Can you work these out from the model? Positions are in its coordinate system, mm. A direction names the side the tool comes from. Give positions to 0.01 mm unless a question says otherwise; leave off trailing zeros. Order: outer loops, then holes, each group sorted by start corner. A loop starts at its lowest first (then second) coordinate and runs counter-clockwise, first axis right, second up. Notation, with made-up numbers: (-10, -3) - (10, -3) arc R35 cw to (10, 32) - close; hole circle Ø8 at (-10.5, 82.5). An arc over 180 degrees is marked (long way). Answer as a JSON object with one key per item and string values.
```python
from build123d import *

# Parameters (mm, degrees)
F0_W      = 155
F0_H      = 80.5
F1_DEPTH  = 8.6
F2_T      = -1.5
F3_W      = 155
F3_H      = 80.5
F3_W_2    = 152
F3_H_2    = 77.5
F3_W_3    = 149
F3_H_3    = 74.5
F4_DEPTH  = 1.5
F5_W      = 28
F5_H      = 7.1
F6_DEPTH  = 1.5
F7_W      = 20
F7_H      = 7.1
F8_DEPTH  = 1.5
F9_R      = 3
F10_DEPTH = 1.5
F11_W     = 38
F11_H     = 6.2492947091
F12_DEPTH = 1.5
F13_W     = 8.8
F13_H     = 4.4
F13_W_2   = 15.4
F13_H_2   = 7.7
F14_DEPTH = 1.5
F15_R     = 1.5
F16_R     = 2
F17_R     = 5
F18_R     = 3
F20_DEPTH = 2
F21_R     = 1.99999
F23_DEPTH = 2
F24_R     = 1.5
F25_DEPTH = 2
F26_R     = 1.5


# Not quite as in the source:
# - a fillet or chamfer is up to 0.001 mm smaller than in the source, because OpenCascade refuses the exact size


with BuildPart() as f1:
    # F0 (on Top) → F1 (new body)
    with BuildSketch(Plane.XY):
        with Locations((77.5, 40.25)):
            Rectangle(F0_W, F0_H)
    extrude(amount=F1_DEPTH)

    # F2
    f2_openings = [f1.faces().sort_by_distance(p)[0] for p in [
        (77.5, 40.25, 8.6),
    ]]
    offset(amount=F2_T, openings=f2_openings)

    # F3 (on face) → F4 (join)
    with BuildSketch(Plane.XY.offset(8.6)):
        with Locations((77.5, 40.25)):
            Rectangle(F3_W, F3_H)
        with Locations((77.5, 40.25)):
            Rectangle(F3_W_2, F3_H_2, mode=Mode.SUBTRACT)
        with Locations((77.5, 40.25)):
            Rectangle(F3_W_2, F3_H_2)
        with Locations((77.5, 40.25)):
            Rectangle(F3_W_3, F3_H_3, mode=Mode.SUBTRACT)
    extrude(amount=F4_DEPTH)

    # F5 (on face) → F6 (cut, through all)
    with BuildSketch(Plane.XZ):
        with Locations((37.5, 5.05)):
            Rectangle(F5_W, F5_H)
    extrude(amount=-F6_DEPTH, mode=Mode.SUBTRACT)

    # F7 (on face) → F8 (cut, through all)
    with BuildSketch(Plane(origin=(0, 80.5, 0), x_dir=(-1, 0, 0), z_dir=(0, 1, 0))):
        with Locations((-48, 5.05)):
            Rectangle(F7_W, F7_H)
    extrude(amount=-F8_DEPTH, mode=Mode.SUBTRACT)

    # F9 (on face) → F10 (cut, through all)
    with BuildSketch(Plane(origin=(0, 0, 0), x_dir=(0, -1, 0), z_dir=(-1, 0, 0))):
        with Locations((-28, 4.5)):
            Circle(F9_R)
    extrude(amount=-F10_DEPTH, mode=Mode.SUBTRACT)

    # F11 (on face) → F12 (cut, through all)
    with BuildSketch(Plane.YZ.offset(155)):
        with Locations((45.2, 4.6246473546)):
            Rectangle(F11_W, F11_H)
    extrude(amount=-F12_DEPTH, mode=Mode.SUBTRACT)

    # F13 (on face) → F14 (cut, through all)
    with BuildSketch(Plane(origin=(0, 0, 0), x_dir=(1, 0, 0), z_dir=(0, 0, -1))):
        with Locations((26.2872223049, -27.05)):
            Rectangle(F13_W, F13_H)
        with Locations((26.2872223049, -22.65)):
            Rectangle(F13_W, F13_H)
        with Locations((26.2872223049, -35.8)):
            Rectangle(F13_W_2, F13_H_2)
        with Locations((26.2872223049, -43.5)):
            Rectangle(F13_W_2, F13_H_2)
        with Locations((26.2872223049, -52.25)):
            Rectangle(F13_W, F13_H)
        with Locations((26.2872223049, -56.65)):
            Rectangle(F13_W, F13_H)
    extrude(amount=-F14_DEPTH, mode=Mode.SUBTRACT)

    # F15
    f15_edges = [f1.edges().sort_by_distance(p)[0] for p in [
        (23.5, 0.75, 8.6),
        (51.5, 0.75, 8.6),
        (51.5, 0.75, 1.5),
        (23.5, 0.75, 1.5),
        (154.25, 26.2, 7.749295),
        (154.25, 26.2, 1.5),
        (154.25, 64.2, 7.749295),
        (154.25, 64.2, 1.5),
        (58, 79.75, 8.6),
        (58, 79.75, 1.5),
        (38, 79.75, 8.6),
        (38, 79.75, 1.5),
        (21.887222, 50.05, 0.75),
    ]]
    fillet(f15_edges, radius=F15_R)

    # F16
    f16_edges = [f1.edges().sort_by_distance(p)[0] for p in [
        (21.887222, 29.25, 0.75),
        (18.587222, 47.35, 0.75),
        (21.887222, 58.85, 0.75),
        (21.887222, 20.45, 0.75),
        (18.587222, 31.95, 0.75),
        (30.687222, 50.05, 0.75),
        (33.987222, 31.95, 0.75),
        (30.687222, 20.45, 0.75),
        (30.687222, 29.25, 0.75),
        (33.987222, 47.35, 0.75),
        (30.687222, 58.85, 0.75),
    ]]
    fillet(f16_edges, radius=F16_R)

    # F17
    f17_edges = [f1.edges().sort_by_distance(p)[0] for p in [
        (0, 0, 5.05),
        (0, 80.5, 5.05),
        (155, 0, 5.05),
        (155, 80.5, 5.05),
    ]]
    fillet(f17_edges, radius=F17_R)

    # F18
    f18_edges = [f1.edges().sort_by_distance(p)[0] for p in [
        (1.5, 79, 5.05),
        (1.5, 1.5, 5.05),
        (153.5, 79, 5.05),
        (153.5, 1.5, 5.05),
    ]]
    fillet(f18_edges, radius=F18_R)

    # F19 (on face) → F20 (join)
    with BuildSketch(Plane(origin=(0, 0, 0), x_dir=(1, 0, 0), z_dir=(0, 0, -1))):
        with BuildLine():
            Line((26.2872223049, -17.0733576864), (12.2872223049, -17.0733576864))
            Line((12.2872223049, -17.0733576864), (12.2872223049, -65.0733576864))
            Line((12.2872223049, -65.0733576864), (26.2872223049, -65.0733576864))
            Line((26.2872223049, -65.0733576864), (26.2872223049, -58.85))
            Line((26.2872223049, -58.85), (23.8872223049, -58.85))
            ThreePointArc((23.8872223049, -58.85), (22.4730087426, -58.2642135624), (21.8872223049, -56.85))
            Line((21.8872223049, -56.85), (21.8872223049, -51.55))
            ThreePointArc((21.8872223049, -51.55), (22.3265621332, -50.4893398282), (23.3872223049, -50.05))
            Line((23.3872223049, -50.05), (26.2872223049, -50.05))
            Line((26.2872223049, -50.05), (26.2872223049, -47.35))
            Line((26.2872223049, -47.35), (20.5872223049, -47.35))
            ThreePointArc((20.5872223049, -47.35), (19.1730087426, -46.7642135624), (18.5872223049, -45.35))
            Line((18.5872223049, -45.35), (18.5872223049, -33.95))
            ThreePointArc((18.5872223049, -33.95), (19.1730087426, -32.5357864376), (20.5872223049, -31.95))
            Line((20.5872223049, -31.95), (26.2872223049, -31.95))
            Line((26.2872223049, -31.95), (26.2872223049, -29.25))
            Line((26.2872223049, -29.25), (23.8872223049, -29.25))
            ThreePointArc((23.8872223049, -29.25), (22.4730087426, -28.6642135624), (21.8872223049, -27.25))
            Line((21.8872223049, -27.25), (21.8872223049, -22.45))
            ThreePointArc((21.8872223049, -22.45), (22.4730087426, -21.0357864376), (23.8872223049, -20.45))
            Line((23.8872223049, -20.45), (26.2872223049, -20.45))
            Line((26.2872223049, -20.45), (26.2872223049, -17.0733576864))
        make_face()
        with BuildLine():
            Line((40.2872223049, -17.0733576864), (26.2872223049, -17.0733576864))
            Line((26.2872223049, -17.0733576864), (26.2872223049, -20.45))
            Line((26.2872223049, -20.45), (28.6872223049, -20.45))
            ThreePointArc((28.6872223049, -20.45), (30.1014358673, -21.0357864376), (30.6872223049, -22.45))
            Line((30.6872223049, -22.45), (30.6872223049, -27.25))
            ThreePointArc((30.6872223049, -27.25), (30.1014358673, -28.6642135624), (28.6872223049, -29.25))
            Line((28.6872223049, -29.25), (26.2872223049, -29.25))
            Line((26.2872223049, -29.25), (26.2872223049, -31.95))
            Line((26.2872223049, -31.95), (31.9872223049, -31.95))
            ThreePointArc((31.9872223049, -31.95), (33.4014358673, -32.5357864376), (33.9872223049, -33.95))
            Line((33.9872223049, -33.95), (33.9872223049, -45.35))
            ThreePointArc((33.9872223049, -45.35), (33.4014358673, -46.7642135624), (31.9872223049, -47.35))
            Line((31.9872223049, -47.35), (26.2872223049, -47.35))
            Line((26.2872223049, -47.35), (26.2872223049, -50.05))
            Line((26.2872223049, -50.05), (28.6872223049, -50.05))
            ThreePointArc((28.6872223049, -50.05), (30.1014358673, -50.6357864376), (30.6872223049, -52.05))
            Line((30.6872223049, -52.05), (30.6872223049, -56.85))
            ThreePointArc((30.6872223049, -56.85), (30.1014358673, -58.2642135624), (28.6872223049, -58.85))
            Line((28.6872223049, -58.85), (26.2872223049, -58.85))
            Line((26.2872223049, -58.85), (26.2872223049, -65.0733576864))
            Line((26.2872223049, -65.0733576864), (40.2872223049, -65.0733576864))
            Line((40.2872223049, -65.0733576864), (40.2872223049, -17.0733576864))
        make_face()
    extrude(amount=F20_DEPTH)

    # F21 (radius 2 in the source; OpenCascade refuses exactly that, so slightly less here)
    f21_edges = [f1.edges().sort_by_distance(p)[0] for p in [
        (12.287222, 17.073358, -1),
        (40.287222, 17.073358, -1),
        (12.287222, 65.073358, -1),
        (40.287222, 65.073358, -1),
        (12.287222, 41.073358, -2),
        (26.287222, 65.073358, -2),
        (40.287222, 41.073358, -2),
        (26.287222, 17.073358, -2),
    ]]
    fillet(f21_edges, radius=F21_R)

    # F22 (on face) → F23 (join)
    with BuildSketch(Plane(origin=(0, 0, 0), x_dir=(1, 0, 0), z_dir=(0, 0, -1))):
        with BuildLine():
            ThreePointArc((139.0328407288, -9.85), (137.2650737758, -10.582233047), (136.5328407288, -12.35))
            Line((136.5328407288, -12.35), (136.5328407288, -40.25))
            Line((136.5328407288, -40.25), (141.5328407288, -40.25))
            Line((141.5328407288, -40.25), (141.5328407288, -12.35))
            ThreePointArc((141.5328407288, -12.35), (140.8006076817, -10.582233047), (139.0328407288, -9.85))
        make_face()
        with BuildLine():
            Line((141.5328407288, -40.25), (136.5328407288, -40.25))
            Line((136.5328407288, -40.25), (136.5328407288, -68.15))
            ThreePointArc((136.5328407288, -68.15), (137.2650737758, -69.917766953), (139.0328407288, -70.65))
            ThreePointArc((139.0328407288, -70.65), (140.8006076817, -69.917766953), (141.5328407288, -68.15))
            Line((141.5328407288, -68.15), (141.5328407288, -40.25))
        make_face()
    extrude(amount=F23_DEPTH)

    # F24
    f24_edges = [f1.edges().sort_by_distance(p)[0] for p in [
        (139.032841, 9.85, -2),
    ]]
    fillet(f24_edges, radius=F24_R)

    # F22 (on face) → F25 (join)
    with BuildSketch(Plane(origin=(0, 0, 0), x_dir=(1, 0, 0), z_dir=(0, 0, -1))):
        with BuildLine():
            ThreePointArc((81.033386401, -10.1015902981), (79.265619448, -10.8338233452), (78.533386401, -12.6015902981))
            Line((78.533386401, -12.6015902981), (78.533386401, -68.4015902981))
            ThreePointArc((78.533386401, -68.4015902981), (79.265619448, -70.1693572511), (81.033386401, -70.9015902981))
            ThreePointArc((81.033386401, -70.9015902981), (82.8011533539, -70.1693572511), (83.533386401, -68.4015902981))
            Line((83.533386401, -68.4015902981), (83.533386401, -12.6015902981))
            ThreePointArc((83.533386401, -12.6015902981), (82.8011533539, -10.8338233452), (81.033386401, -10.1015902981))
        make_face()
    extrude(amount=F25_DEPTH)

    # F26
    f26_edges = [f1.edges().sort_by_distance(p)[0] for p in [
        (78.533386, 40.50159, -2),
    ]]
    fillet(f26_edges, radius=F26_R)


solid = f1.part
```
Q1. Which directions (+Z, -Z, +X, -X, +Y, -Y) give clear straight access to the entire face, cutting with the end or side of a thin tool? Please do faces 1 (the face through (72, 2, 8.6)), 2 (the face through (18, 41, -2)), 3 (the face through (0.7, 31, 4.6)), 4 (the face through (26, 29.25, 0)).
Recorded:
{"face 1": "none", "face 2": "-Z, +X, -X, +Y, -Y", "face 3": "-X", "face 4": "+Z, -Z"}
Q2. We'd pull the mould along X, two halves only. Please class faces 5 (the face through (153.5, 79.07, 4.98)), 6 (the face through (1.43, 79, 4.98)), 7 (the face through (26, 47.35, 0)): released by +X, released by -X, zero draft, split by the parting line, or undercut.
Recorded:
{"face 5": "released by +X", "face 6": "released by -X", "face 7": "undercut"}
Q3. I'm going to push flat-ended pins straight in: pin 1 Ø12 at (x, y) = (61, 33) entering from -Z; pin 2 Ø1.5 at (x, y) = (17.5, 64.5) entering from +Z; pin 3 Ø1.2 at (x, z) = (154.5, 4) entering from -Y. Where does each tip first touch, or does it pass through?
Recorded:
{"pin 1": "stops at z = 0", "pin 2": "stops at z = 1.5", "pin 3": "stops at y = 1.87"}
Q4. If we section it at A-A, the plane z = 4.5: Count the separate pieces of the cut face and the enclosed holes in it, then the cut area to 3 significant figures.
Recorded:
{"separate pieces": "4", "enclosed holes": "0", "area": "546 mm^2"}
Q5. If we section it at B-B, the plane x = 97: Please give me the cut outline in (y, z), then the cut area to 3 significant figures.
Recorded:
{"outline": "(0, 0) - (80.5, 0) - (80.5, 10.1) - (77.5, 10.1) - (77.5, 8.6) - (79, 8.6) - (79, 1.5) - (1.5, 1.5) - (1.5, 8.6) - (3, 8.6) - (3, 10.1) - (0, 10.1) - close", "area": "151 mm^2"}
Q6. I need wall thicknesses on L1, parallel to Z at x = 0.5, y = 28; L2, parallel to X at y = 64.5, z = 7.25; L3, parallel to Y at x = 16, z = 3.75. Which ranges of each line are inside material? Lowest first, please.
Recorded:
{"L1": "z = 0 to 1.5, 7.5 to 10.1", "L2": "x = 0 to 1.5, 153.5 to 155", "L3": "y = 0 to 1.5, 79 to 80.5"}
